Input: part model. Units: mm. Frame: model coordinates. A direction names the side the tool comes from. Give positions to 0.01 mm unless a question says otherwise; leave off trailing zeros. Loops run counter-clockwise (first coordinate to the right, second up) from the corner with the lowest first, then second, coordinate; pieces in that order, holes last. Notation, with made-up numbers: M 14,57 L 33,57 A6 cw 33,61 Z; hole C -10,83.25 d7. An arc over 180 degrees is marked long. One line per item, written item: value. Start each with the question number.
(1) Section A-A on x = 55. Output: boundary loops of the cut face in (y, z), plus the area to 3 significant figures.
(2) Pin query (flat end, axial travel): P1, Ø7.5, axis at x = 64, z = 15, coming from the -Y side; P2, Ø16.5, axis at x = 53.5, y = -12.5, coming from the -Z side; P3, Ø12, axis at y = -18.5, z = 22.5, coming from the +X side. Return the tip coordinate at first contact, or that it passes through.
(3) Ray query, line 1 along Y through (x, z) = (71, 2); line 2 along Z through (x, y) = (97.5, -8); line 3 along Z through (x, y) = (57, -33.5). Return the intervals inside material, ascending. Write a range as from..to.
(4) Section B-B on y = -2. Output: boundary loops of the cut face in (x, z), plus the area to 3 significant figures.
(5) Access query for faces 1 (the flat face through (56, 0, 13)), 2 (the flat face through (56, 2, 0)). Directions: +Z, -Z, +X, -X, +Y, -Y. A direction counts if a zero-diameter tool reaches every point of the face in a straight line with its end or side. Return the directions, or none.
(6) Section C-C on z = 22. Output: boundary loops of the cut face in (x, y), plus the area to 3 significant figures.
```python
from build123d import *

# Parameters (mm, degrees)
F1_DEPTH = 114.3
F3_DEPTH = 41.149
F4_SIZE2 = 1.848969
F4_SIZE  = 5.08


with BuildPart() as f1:
    # F0 (on Right) → F1 (new body)
    with BuildSketch(Plane.YZ):
        Polygon((0, 25.4), (0, 0), (3.048, 0), (3.048, 27.94), (-38.1, 27.94), (-38.1, 25.4), align=None)
    extrude(amount=F1_DEPTH)

    # F2 (on face) → F3 (cut, through all)
    with BuildSketch(Plane(origin=(0, 3.048, 0), x_dir=(-1, 0, 0), z_dir=(0, 1, 0))):
        Polygon((-107.95, 0), (-114.3, 27.94), (-114.3, 0), align=None)
        Polygon((0, 0), (0, 27.94), (-6.35, 0), align=None)
    extrude(amount=-F3_DEPTH, mode=Mode.SUBTRACT)

    # F4
    f4_edges = [f1.edges().sort_by_distance(p)[0] for p in [
        (57.15, -38.1, 25.4),
    ]]
    chamfer(f4_edges, length=F4_SIZE, length2=F4_SIZE2)


solid = f1.part
```
Output values:
1. outline: M -38.1,27.25 L -33.02,25.4 L 0,25.4 L 0,0 L 3.05,0 L 3.05,27.94 L -38.1,27.94 Z
1. area: 177 mm²
2. P1: stops at y = 0
2. P2: stops at z = 25.4
2. P3: stops at x = 114.3
3. line 1: y = 0..3.05
3. line 2: z = 25.4..27.94
3. line 3: z = 25.57..27.94
4. outline: M 0,27.94 L 0.58,25.4 L 113.72,25.4 L 114.3,27.94 Z
4. area: 289 mm²
5. face 1: -Z, +X, -X, -Y
5. face 2: -Z, +X, -X, +Y, -Y
6. outline: M 1.35,0 L 112.95,0 L 112.95,3.05 L 1.35,3.05 Z
6. area: 340 mm²
